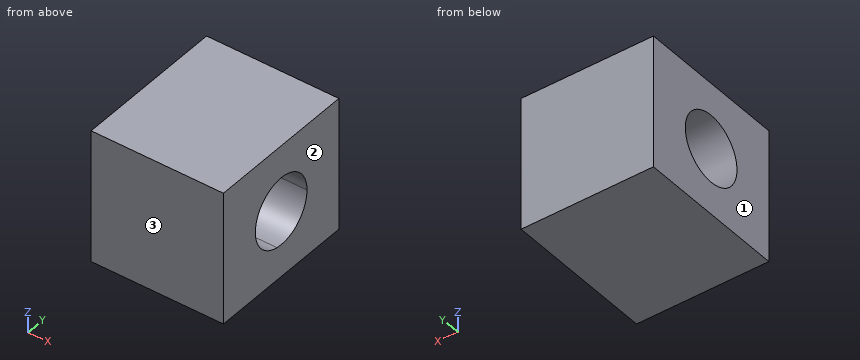
```python
from build123d import *

# Parameters (mm, degrees)
F0_W     = 73.074155
F0_H     = 63.90892
F1_DEPTH = 63.5
F3_DEPTH = 63.5


with BuildPart() as f1:
    # F0 (on Right) → F1 (new body)
    with BuildSketch(Plane.YZ):
        with Locations((36.537077, 31.95446)):
            Rectangle(F0_W, F0_H)
    extrude(amount=F1_DEPTH)

    # F2 (on face) → F3 (cut)
    with BuildSketch(Plane.YZ.offset(63.5)):
        with BuildLine():
            ThreePointArc((24.867562, 20.489157), (29.021198, 17.423723), (33.923234, 15.8052))
            ThreePointArc((33.923234, 15.8052), (30.073151, 19.457503), (24.867562, 20.489157))
        make_face()
        with BuildLine():
            ThreePointArc((24.867562, 20.489157), (30.073151, 19.457503), (33.923234, 15.8052))
            ThreePointArc((33.923234, 15.8052), (47.14061, 19.496697), (52.896502, 31.95446))
            ThreePointArc((52.896502, 31.95446), (30.343362, 47.09608), (24.867562, 20.489157))
        make_face()
    extrude(amount=-F3_DEPTH, mode=Mode.SUBTRACT)


solid = f1.part
```
Input: part model. Units: mm. Frame: model coordinates. Face numbers are marked on the shaded views. Give positions to 0.01 mm unless a question says otherwise; leave off trailing zeros. Order: outer loops, then holes, each group sorted by start corner. A loop starts at its lowest first (then second) coordinate and runs counter-clockwise, first axis right, second up.
1. Material intervals for L1, parallel to Z at x = 44, y = 40; L2, parallel to Y at x = 52.5, z = 39; L3, parallel to Y at x = 32, z = 26, sorted ascending.
Derived:
L1: z = 0 to 15.97, 47.94 to 63.91
L2: y = 0 to 21.77, 51.3 to 73.07
L3: y = 0 to 21.3, 51.77 to 73.07
2. Section A-A on z = 35.5. Return the cut outline in (x, y).
Derived:
outline: (0, 0) - (63.5, 0) - (63.5, 20.57) - (0, 20.57) - close; (0, 52.51) - (63.5, 52.51) - (63.5, 73.07) - (0, 73.07) - close
3. Mould query, pull axis X, two halves, no side actions, for the marked faces 1, 2 and 3. Classes: released by +X, released by -X, zero draft, split by the parting line, or undercut.
Derived:
face 1: released by -X
face 2: released by +X
face 3: zero draft
4. Pin query (flat end, axial travel): pin 1 (8 mm diameter, centred on y = 32.5, z = 49.5, fed in from -X). Return the tip coordinate at first contact, or that it passes through.
Derived:
pin 1: stops at x = 0
5. Section B-B on y = 28.5. Return the cut outline in (x, z), and give its area (3 significant figures).
Derived:
outline: (0, 0) - (63.5, 0) - (63.5, 17.71) - (0, 17.71) - close; (0, 46.2) - (63.5, 46.2) - (63.5, 63.91) - (0, 63.91) - close
area: 2,250 mm2
6. Section C-C on x = 50. Return the cut outline in (y, z).
Derived:
outline: (0, 0) - (73.07, 0) - (73.07, 63.91) - (0, 63.91) - close; hole (24.87, 20.49) arc R16.36 ccw to (33.92, 15.81) arc R16.36 ccw (long way) to start
